Verification items for the finished model (mm, model axes). Give positions to 0.01 mm unless a question says otherwise; leave off trailing zeros. Write each loop counter-clockwise with the first axis right and the second up, starting at its lowest first coordinate (ties: lowest second). Pieces come first, ordered by that corner, then holes. Notation, with made-up numbers: (-26.5, 1.5) -> (-7.5, 1.5) arc R32 ccw to (-7.5, 31.5) -> close; hole circle Ø2 at (57.5, -8). An arc over 180 degrees is marked (long way). Answer as CSV lines item,"result".
Autodesk Inventor part; units mm, degrees
ref_plane "YZ Plane" through (0, 0, 0) normal (1, 0, 0) x (0, 1, 0)
ref_plane "XZ Plane" through (0, 0, 0) normal (0, 1, 0) x (-1, 0, 0)
ref_plane "XY Plane" through (0, 0, 0) normal (0, 0, 1) x (1, 0, 0)
sketch "草图1" plane through (0, 0, 0) normal (0, 0, 1) x (1, 0, 0)
  line L0 (18.5, -15.5) -> (-18.5, -15.5)
  line L1 (-18.5, -15.5) -> (-18.5, 15.5)
  line L2 (-18.5, 15.5) -> (18.5, 15.5)
  line L3 (18.5, 15.5) -> (18.5, -15.5)
  line L4 (18.5, -15.5) -> (-18.5, 15.5) construction
  line L5 (-18.5, -15.5) -> (18.5, 15.5) construction
  line L6 (0, 0) -> (-24.9379, 0) construction
  line L7 (0, 0) -> (0, 16.8364) construction
  point P0 (-15, 12)
  point P1 (-15, -12)
  point P2 (15, 12)
  point P3 (15, -12)
  dimension "d0" = 31
  dimension "d1" = 37
  dimension "d2" = 12
  dimension "d3" = 15
extrude "拉伸1" add sketch "草图1" along normal blind 0.5
hole "孔1" at (-15, 12, 0) at (-15, -12, 0) at (15, 12, 0) at (15, -12, 0) direction (0, 0, 1) diameter 4.2 end through all
properties part number "自制垫片"
1) Depth check by flat-ended pin: pin 1 (3.5 mm diameter, centred on x = -15, y = 12, fed in from +Z). Enter the tip coordinate at first touch or a pass-through.
Reported:
pin 1,"through"
2) Section check B-B (z = 0.1). Record the boundary of the cut face in (x, y).
Reported:
outline,"(-18.5, -15.5) -> (18.5, -15.5) -> (18.5, 15.5) -> (-18.5, 15.5) -> close; hole circle Ø4.2 at (-15, -12); hole circle Ø4.2 at (-15, 12); hole circle Ø4.2 at (15, -12); hole circle Ø4.2 at (15, 12)"
3) Draft check along Y on faces 1 (the flat face through (0, 0, 0.5)), 2 (the cylindrical face through (-16.419, -13.548, 0.254)), 3 (the cylindrical face through (12.918, 11.727, 0.254)). Enter one of: +Y half, -Y half, draft (parallel to the pull), parting line (faces both ways), or undercut.
Reported:
face 1,"draft"
face 2,"undercut"
face 3,"undercut"
4) Scan lines: line 1 along Y through (x, z) = (-15, 0.2); line 2 along X through (y, z) = (-12, 0.1); line 3 along X through (y, z) = (-10.5, 0.45). Record each from-to range of solid material in increasing order.
Reported:
line 1,"-15.5 to -14.1, -9.9 to 9.9, 14.1 to 15.5"
line 2,"-18.5 to -17.1, -12.9 to 12.9, 17.1 to 18.5"
line 3,"-18.5 to -16.47, -13.53 to 13.53, 16.47 to 18.5"
5) Section check C-C (x = -15). Record the boundary of the cut face in (y, z).
Reported:
outline,"(-15.5, 0) -> (-14.1, 0) -> (-14.1, 0.5) -> (-15.5, 0.5) -> close; (-9.9, 0) -> (9.9, 0) -> (9.9, 0.5) -> (-9.9, 0.5) -> close; (14.1, 0) -> (15.5, 0) -> (15.5, 0.5) -> (14.1, 0.5) -> close"
6) Section check A-A (y = -12). Record the boundary of the cut face in (x, z).
Reported:
outline,"(-18.5, 0) -> (-17.1, 0) -> (-17.1, 0.5) -> (-18.5, 0.5) -> close; (-12.9, 0) -> (12.9, 0) -> (12.9, 0.5) -> (-12.9, 0.5) -> close; (17.1, 0) -> (18.5, 0) -> (18.5, 0.5) -> (17.1, 0.5) -> close"
